Part print with two shaded views. Sizes in mm from the minimum x, y, z corner. A direction names the side the tool comes from. Give positions to 0.01 mm unless a question says otherwise; leave off trailing zeros. Write each loop counter-clockwise with the first axis right and the second up, starting at its lowest first coordinate (ties: lowest second). Pieces come first, ordered by that corner, then holes. Notation, with made-up numbers: (27, 79.5) - (46, 79.5) arc R28 cw to (46, 100.5) - close; hole circle Ø3 at (62, 25). An arc over 180 degrees is marked (long way). One line per item, written item: value. Start each with the question number.
(1) Cut at B-B, the plane z = 1.75. List the corners of the cut face in (x, y), and give its area (3 significant figures).
(2) Cut at A-A, the plane x = 23. List the corners of the cut face in (y, z), and give its area (3 significant figures).
(3) Drop flat-ended pins along their axis: P1, Ø5, axis at x = 26, z = 6.5, coming from the +Y side; P2, Ø3, axis at y = 15, z = 6.5, coming from the -X side; P3, Ø6, axis at x = 5.5, y = 23, coming from the +Z side. Give the stop position or say it passes through.
(4) Probe L1, parallel to Y at x = 23, z = 6.8; L2, parallel to Z at x = 43, y = 29. List the from-to ranges inside material, lowest first.
(5) 3-axis set-ups, long thin cutter, end or side, ignore diameter. For the marked faces 4, 5 and 6: which of +Z, -Z, +X, -X, +Y, -Y reach the whole face in a straight line?
(6) Cut at D-D, the plane y = 5.5. List the corners of the cut face in (x, z), and give its area (3 significant figures).
(7) Mould opens along X. For the marked faces 1, 2 and 3 say: pulls with the +X half, pulls with the -X half, needs draft (parallel to the pull), parting line crosses it, or undercut.
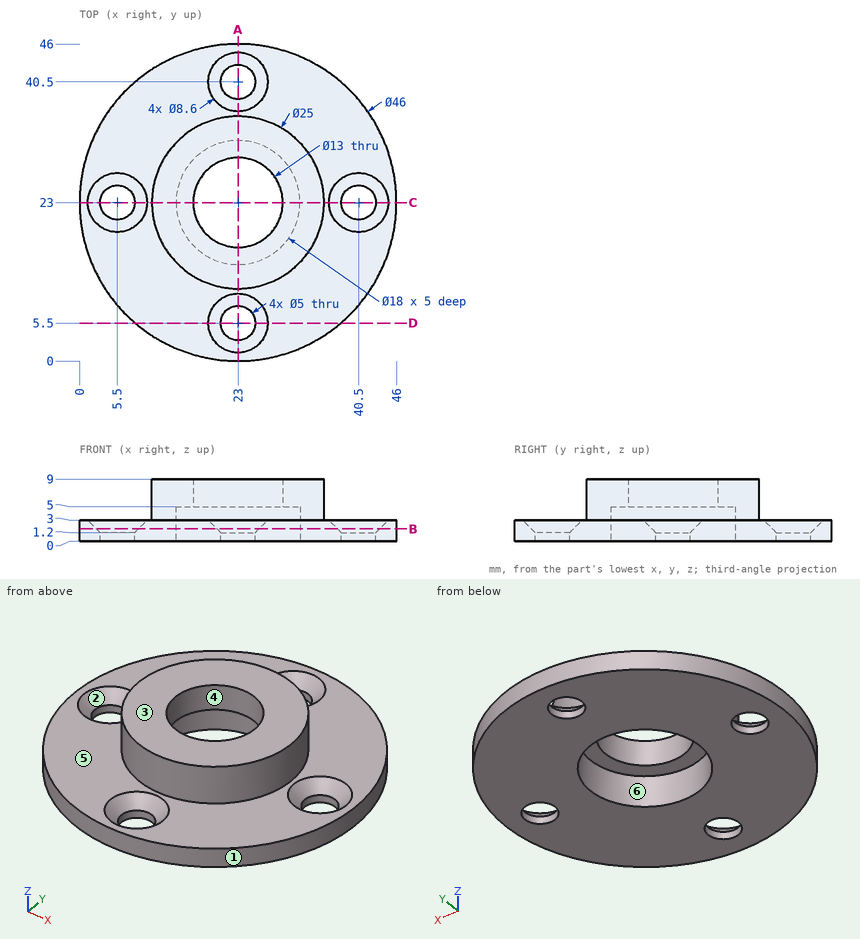
Answers follow:
1. outline: circle Ø46 at (23, 23); hole circle Ø6.1 at (5.5, 23); hole circle Ø18 at (23, 23); hole circle Ø6.1 at (23, 5.5); hole circle Ø6.1 at (23, 40.5); hole circle Ø6.1 at (40.5, 23)
1. area: 1,290 mm²
2. outline: (0, 0) - (3, 0) - (3, 1.2) - (1.2, 3) - (0, 3) - close; (8, 0) - (14, 0) - (14, 5) - (16.5, 5) - (16.5, 9) - (10.5, 9) - (10.5, 3) - (9.8, 3) - (8, 1.2) - close; (29.5, 5) - (32, 5) - (32, 0) - (38, 0) - (38, 1.2) - (36.2, 3) - (35.5, 3) - (35.5, 9) - (29.5, 9) - close; (43, 0) - (46, 0) - (46, 3) - (44.8, 3) - (43, 1.2) - close
2. area: 110 mm²
3. P1: stops at y = 35.49
3. P2: stops at x = 12.32
3. P3: stops at z = 1.7
4. L1: y = 10.5 to 16.5, 29.5 to 35.5
4. L2: z = 0 to 3
5. face 4: +Z, -Z
5. face 5: +Z
5. face 6: -Z
6. outline: (8.08, 0) - (20.5, 0) - (20.5, 1.2) - (18.7, 3) - (8.08, 3) - close; (25.5, 0) - (37.92, 0) - (37.92, 3) - (27.3, 3) - (25.5, 1.2) - close
6. area: 71.3 mm²
7. face 1: parting line crosses it
7. face 2: undercut
7. face 3: needs draft
